Geometry check sheet. Reference: the model listing, model coordinates, mm. A direction names the side the tool comes from. Round coordinates to 2 decimals unless told otherwise and drop trailing zeros. Order: outer loops, then holes, each group sorted by start corner. A loop starts at its lowest first (then second) coordinate and runs counter-clockwise, first axis right, second up.
(1) Cross-section at C-C on z = 5. Enter the section's corners in (x, y), and give its area (3 significant figures).
(2) Set-up check for faces 1 (the face through (-11, 4, 2.273)), 2 (the face through (0, 4, -9.525)), 3 (the face through (12.69, 4.2, -1.7)), 4 (the face through (-9.49, 4.2, -8.95)): record each of +Z, -Z, +X, -X, +Y, -Y from which the full face is reachable in a straight line by a thin tool's end or side.
(3) Thickness scan on L1, parallel to Y at x = -0.5, z = -11.5; L2, parallel to Y at x = -9, z = -3.5; L3, parallel to Z at x = -4.5, y = 5.5 (3 decimals). Record the ranges inside material, lowest first.
(4) Cross-section at A-A on x = 0. Enter the section's corners in (y, z) (3 decimals), and give its area (3 significant figures).
(5) Cross-section at D-D on y = 20.25. Enter the section's corners in (x, z), and give its area (3 significant figures).
(6) Cross-section at B-B on y = 3. Enter the section's corners in (x, z) (3 decimals).
(7) Gauge pin test, flat ends, axial feed: P1, Ø1, axis at x = 1, y = 9.5, coming from the -Z side; P2, Ø1.5, axis at x = 0.5, y = 5.5, coming from the +Z side (3 decimals); P3, Ø2.5, axis at x = 1.5, y = 4.5, coming from the -Z side (3 decimals). Record the tip position at first contact, or that the pin passes through.
from build123d import *

# Parameters (mm, degrees)
SKETCH1_W           = 32
SKETCH1_H           = 32
SKETCH1_R           = 1.04775
BOSS_EXTRUDE1_DEPTH = 1.6002
BOSS_EXTRUDE2_DEPTH = 5.1308
FILLET1_R           = 2.1
FILLET2_R           = 1.905
SKETCH3_R           = 7.5946
BOSS_EXTRUDE3_DEPTH = 16.129


with BuildPart() as part:
    # Sketch1 → Boss-Extrude1 (new body)
    with BuildSketch(Plane(origin=(0, 0, 0), x_dir=(1, 0, 0), z_dir=(0, 1, 0))):
        Rectangle(SKETCH1_W, SKETCH1_H)
        with Locations(Location((13.7500106, 13.7500106, 0), (0, 0, 270))):
            Circle(SKETCH1_R, mode=Mode.SUBTRACT)
        with Locations(Location((-13.7500106, 13.7500106, 0), (0, 0, 270))):
            Circle(SKETCH1_R, mode=Mode.SUBTRACT)
        with Locations(Location((-13.75, -13.7500106, 0), (0, 0, 270))):
            Circle(SKETCH1_R, mode=Mode.SUBTRACT)
        with Locations(Location((13.7500106, -13.7500106, 0), (0, 0, 270))):
            Circle(SKETCH1_R, mode=Mode.SUBTRACT)
    extrude(amount=BOSS_EXTRUDE1_DEPTH)

    # Sketch2 → Boss-Extrude2 (add)
    with BuildSketch(Plane(origin=(0, 1.6002, 0), x_dir=(1, 0, 0), z_dir=(0, 1, 0))):
        Polygon((-10.033, 9.525), (10.033, 9.525), (10.033, 2.2733), (13.2334, 2.2733), (13.2334, -2.2733), (10.033, -2.2733), (10.033, -9.525), (-10.033, -9.525), (-10.033, -2.2733), (-13.2334, -2.2733), (-13.2334, 2.2733), (-10.033, 2.2733), align=None)
    extrude(amount=BOSS_EXTRUDE2_DEPTH)

    # Fillet1
    fillet1_edges = [part.edges().sort_by_distance(p)[0] for p in [
        (-16, 0.8001, -16),
        (16, 0.8001, -16),
        (16, 0.8001, 16),
        (-16, 0.8001, 16),
    ]]
    fillet(fillet1_edges, radius=FILLET1_R)

    # Fillet2
    fillet2_edges = [part.edges().sort_by_distance(p)[0] for p in [
        (-10.033, 4.1656, -9.525),
        (-13.2334, 4.1656, -2.2733),
        (-13.2334, 4.1656, 2.2733),
        (-10.033, 4.1656, 9.525),
        (10.033, 4.1656, 9.525),
        (13.2334, 4.1656, 2.2733),
        (13.2334, 4.1656, -2.2733),
        (10.033, 4.1656, -9.525),
    ]]
    fillet(fillet2_edges, radius=FILLET2_R)

    # Sketch3 → Boss-Extrude3 (add)
    with BuildSketch(Plane(origin=(0, 6.731, 0), x_dir=(1, 0, 0), z_dir=(0, 1, 0))):
        with Locations(Location((0, 0, 0), (0, 0, 90))):
            Circle(SKETCH3_R)
    extrude(amount=BOSS_EXTRUDE3_DEPTH)


solid = part.part
Found:
1. outline: (-16, 0) - (16, 0) - (16, 1.6) - (10.03, 1.6) - (10.03, 6.73) - (5.72, 6.73) - (5.72, 22.86) - (-5.72, 22.86) - (-5.72, 6.73) - (-10.03, 6.73) - (-10.03, 1.6) - (-16, 1.6) - close
1. area: 339 mm2
2. face 1: +Z, -X, +Y
2. face 2: -Z, +X, -X, +Y
2. face 3: -Z, +X, +Y
2. face 4: -Z, -X, +Y
3. L1: y = 0 to 1.6
3. L2: y = 0 to 6.73
3. L3: z = -9.525 to 9.525
4. outline: (0, -16) - (1.6, -16) - (1.6, -9.525) - (6.731, -9.525) - (6.731, -7.595) - (22.86, -7.595) - (22.86, 7.595) - (6.731, 7.595) - (6.731, 9.525) - (1.6, 9.525) - (1.6, 16) - (0, 16) - close
4. area: 394 mm2
5. outline: circle Ø15.19 at (0, 0)
5. area: 181 mm2
6. outline: (-13.233, -0.368) arc R1.905 ccw to (-11.328, -2.273) - (-10.033, -2.273) - (-10.033, -7.62) arc R1.905 ccw to (-8.128, -9.525) - (8.128, -9.525) arc R1.905 ccw to (10.033, -7.62) - (10.033, -2.273) - (11.328, -2.273) arc R1.905 ccw to (13.233, -0.368) - (13.233, 0.368) arc R1.905 ccw to (11.328, 2.273) - (10.033, 2.273) - (10.033, 7.62) arc R1.905 ccw to (8.128, 9.525) - (-8.128, 9.525) arc R1.905 ccw to (-10.033, 7.62) - (-10.033, 2.273) - (-11.328, 2.273) arc R1.905 ccw to (-13.233, 0.368) - close
7. P1: stops at z = -7.58
7. P2: stops at z = 9.525
7. P3: stops at z = -9.525
